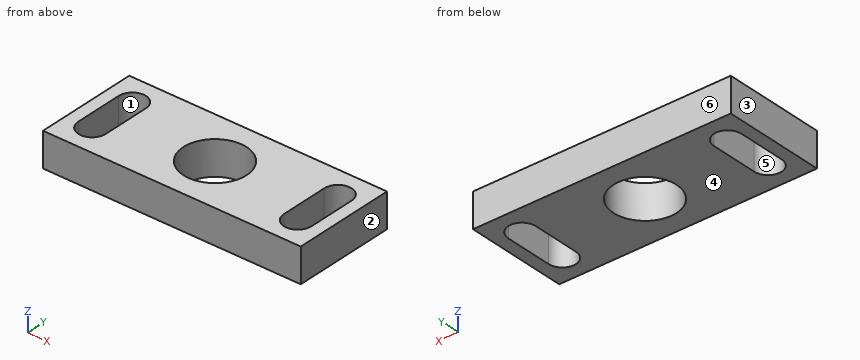
from build123d import *

# Parameters (mm, degrees)
SKETCH1_W           = 37.6
SKETCH1_H           = 15
BOSS_EXTRUDE1_DEPTH = 5
CUT_EXTRUDE1_DEPTH  = 5
SKETCH3_R           = 4.6
CUT_EXTRUDE2_DEPTH  = 5


with BuildPart() as part:
    # Sketch1 → Boss-Extrude1 (new body)
    with BuildSketch(Plane.XY):
        Rectangle(SKETCH1_W, SKETCH1_H)
    extrude(amount=BOSS_EXTRUDE1_DEPTH)

    # Sketch2 → Cut-Extrude1 (cut)
    with BuildSketch(Plane.XY.offset(5)):
        with BuildLine():
            Line((-13, 3.5), (-13, -3.5))
            ThreePointArc((-13, -3.5), (-15, -5.5), (-17, -3.5))
            Line((-17, -3.5), (-17, 3.5))
            ThreePointArc((-17, 3.5), (-15, 5.5), (-13, 3.5))
        make_face()
        with BuildLine():
            Line((17, 3.5), (17, -3.5))
            ThreePointArc((17, -3.5), (15, -5.5), (13, -3.5))
            Line((13, -3.5), (13, 3.5))
            ThreePointArc((13, 3.5), (15, 5.5), (17, 3.5))
        make_face()
    extrude(amount=-CUT_EXTRUDE1_DEPTH, mode=Mode.SUBTRACT)

    # Sketch3 → Cut-Extrude2 (cut)
    with BuildSketch(Plane.XY.offset(5)):
        Circle(SKETCH3_R)
    extrude(amount=-CUT_EXTRUDE2_DEPTH, mode=Mode.SUBTRACT)


solid = part.part
Read the model definition and answer for the solid it produces. Units are mm, in the model's axes. Face numbers are marked on the shaded views. A direction names the side the tool comes from. Coordinates: 2 decimals unless noted, no trailing zeros. Loops run counter-clockwise (first coordinate to the right, second up) from the corner with the lowest first, then second, coordinate; pieces in that order, holes last.
Q1. Consider probe 1 along Y at (x, z) = (0, 2.95); probe 2 along X at (y, z) = (-5, 4.25); probe 3 along X at (y, z) = (-3.5, 4.3). Determine where each line is inside the solid, lowest interval first.
Q2. The part is cut by section D-D on x = 0. Write down the section's boundary in (y, z), and give its area (3 significant figures).
Q3. The part is cut by section C-C on y = 0. Write down the section's boundary in (x, z).
Q4. The part is cut by section B-B on z = 1.55. Write down the section's boundary in (x, y), and give its area (3 significant figures).
Q5. The mould has two halves that part along X. Classify the marked faces 1, 2, 3 and 4: +X half, -X half, draft (parallel to the pull), parting line (faces both ways), or undercut.
Q6. Which of the six approach directions +Z, -Z, +X, -X, +Y, -Y give full straight-line access (tool end or side, diameter ignored) to the marked faces 5 and 6?
Q7. The part is cut by section A-A on x = -15. Write down the section's boundary in (y, z).
Results below:
1. probe 1: y = -7.5 to -4.6, 4.6 to 7.5
1. probe 2: x = -18.8 to -16.32, -13.68 to 13.68, 16.32 to 18.8
1. probe 3: x = -18.8 to -17, -13 to -2.98, 2.98 to 13, 17 to 18.8
2. outline: (-7.5, 0) - (-4.6, 0) - (-4.6, 5) - (-7.5, 5) - close; (4.6, 0) - (7.5, 0) - (7.5, 5) - (4.6, 5) - close
2. area: 29.0 mm2
3. outline: (-18.8, 0) - (-17, 0) - (-17, 5) - (-18.8, 5) - close; (-13, 0) - (-4.6, 0) - (-4.6, 5) - (-13, 5) - close; (4.6, 0) - (13, 0) - (13, 5) - (4.6, 5) - close; (17, 0) - (18.8, 0) - (18.8, 5) - (17, 5) - close
4. outline: (-18.8, -7.5) - (18.8, -7.5) - (18.8, 7.5) - (-18.8, 7.5) - close; hole (-17, -3.5) arc R2 ccw to (-13, -3.5) - (-13, 3.5) arc R2 ccw to (-17, 3.5) - close; hole circle Ø9.2 at (0, 0); hole (13, -3.5) arc R2 ccw to (17, -3.5) - (17, 3.5) arc R2 ccw to (13, 3.5) - close
4. area: 416 mm2
5. face 1: undercut
5. face 2: +X half
5. face 3: -X half
5. face 4: draft
6. face 5: +Z, -Z
6. face 6: +Z, -Z, +X, -X, +Y
7. outline: (-7.5, 0) - (-5.5, 0) - (-5.5, 5) - (-7.5, 5) - close; (5.5, 0) - (7.5, 0) - (7.5, 5) - (5.5, 5) - close
